from build123d import *

# Parameters (mm, degrees)
SKETCH_W        = 18
SKETCH_H        = 10
PAD_DEPTH       = 17
SKETCH009_R     = 1.5
POCKET_DEPTH    = 4
POCKET001_DEPTH = 2.5
POCKET002_DEPTH = 10.001
SKETCH012_R     = 1.5
POCKET003_DEPTH = 10.001


with BuildPart() as part:
    # Sketch → Pad (new body)
    with BuildSketch(Plane.XY):
        with Locations((9, 5)):
            Rectangle(SKETCH_W, SKETCH_H)
    extrude(amount=PAD_DEPTH)

    # Sketch009 (on DatumPlane) → Pocket (cut, symmetric)
    with BuildSketch(Plane.XY.offset(13)):
        with Locations((3, 5)):
            Circle(SKETCH009_R)
        with Locations((15, 5)):
            Circle(SKETCH009_R)
    extrude(amount=POCKET_DEPTH, both=True, mode=Mode.SUBTRACT)

    # Sketch010 (on DatumPlane) → Pocket001 (cut)
    with BuildSketch(Plane.XY.offset(13)):
        Polygon((4.732051, 2), (6.464102, 5), (4.732051, 8), (1.267949, 8), (0, 8), (0, 2), (1.267949, 2), align=None)
        Polygon((16.732051, 8), (13.267949, 8), (11.535898, 5), (13.267949, 2), (16.732051, 2), (18, 2), (18, 8), align=None)
    extrude(amount=-POCKET001_DEPTH, mode=Mode.SUBTRACT)

    # Sketch011 → Pocket002 (cut, through all)
    with BuildSketch(Plane.XZ):
        Polygon((6.45, 0), (11.55, 0), (13.917136, 4.1), (4.082864, 4.1), align=None)
    extrude(amount=-POCKET002_DEPTH, mode=Mode.SUBTRACT)

    # Sketch012 → Pocket003 (cut, through all)
    with BuildSketch(Plane.XZ):
        with Locations((9, 10)):
            Circle(SKETCH012_R)
    extrude(amount=-POCKET003_DEPTH, mode=Mode.SUBTRACT)


solid = part.part
Design review of the part built by this model. Coordinates are the model's own, in mm. A direction names the side the tool comes from. Coordinates: 2 decimals unless noted, no trailing zeros. Loops run counter-clockwise (first coordinate to the right, second up) from the corner with the lowest first, then second, coordinate; pieces in that order, holes last.
Item 1: Add section A-A (z = 10). Write out the cut boundary in (x, y).
Completed:
outline: (0, 0) - (7.5, 0) - (7.5, 10) - (0, 10) - close; (10.5, 0) - (18, 0) - (18, 10) - (10.5, 10) - close; hole circle Ø3 at (3, 5); hole circle Ø3 at (15, 5)
Item 2: For faces 1 (the flat face through (16.2, 6.4, 13)), 2 (the cylindrical face through (4.386, 4.425, 14.972)), 3 (the flat face through (5.25, 4.93, 2.08)), 4 (the flat face through (1.8, 3.7, 13)), list the 3-axis set-ups (+Z, -Z, +X, -X, +Y, -Y) from which the entire face can be reached by the end or side of a thin tool; tool diameter is ignored.
Completed:
face 1: +X
face 2: +Z
face 3: +Y, -Y
face 4: -X
Item 3: Add section B-B (y = 4.5). Give the number of separate pieces and of enclosed holes in the cut face, and give its area (3 significant figures).
Completed:
separate pieces: 3
enclosed holes: 1
area: 206 mm2
Item 4: Add section C-C (x = 9). Write out the cut boundary in (y, z).
Completed:
outline: (0, 4.1) - (10, 4.1) - (10, 8.5) - (0, 8.5) - close; (0, 11.5) - (10, 11.5) - (10, 17) - (0, 17) - close
Item 5: Add section D-D (z = 12.75). Write out the cut boundary in (x, y), and give its area (3 significant figures).
Completed:
outline: (0, 0) - (18, 0) - (18, 2) - (13.27, 2) - (11.54, 5) - (13.27, 8) - (18, 8) - (18, 10) - (0, 10) - (0, 8) - (4.73, 8) - (6.46, 5) - (4.73, 2) - (0, 2) - close
area: 113 mm2
Item 6: Clearance check with flat-ended pins moving along their axes: pin 1 (1.8 mm diameter, centred on x = 9, z = 10, fed in from -Y); pin 2 (2.5 mm diameter, centred on x = 15, y = 5, fed in from +Z); pin 3 (2 mm diameter, centred on x = 8, y = 8, fed in from -Z). State where each tip first meets the part, or that it passes through.
Completed:
pin 1: passes through
pin 2: stops at z = 9
pin 3: stops at z = 4.1
Item 7: Wall thickness on L1, parallel to Y at x = 15, z = 9.85; L2, parallel to Z at x = 12.75, y = 5.75; L3, parallel to Z at x = 2.5, y = 7.25: over which ranges is each line inside the solid? List them lowest first.
Completed:
L1: y = 0 to 3.5, 6.5 to 10
L2: z = 0 to 2.08, 4.1 to 10.5, 13 to 17
L3: z = 0 to 10.5, 13 to 17
Item 8: Draft analysis for pull direction Z (two halves, no side actions). For faces 5 (the flat face through (3, 5, 9)), 6 (the flat face through (9, 5, 4.1)), 7 (the cylindrical face through (13.5, 5.07, 15.03)), 8 (the flat face through (12.717, 4.93, 2.021)), state which applies: pulls with the +Z half, pulls with the -Z half, needs draft (parallel to the pull), parting line crosses it, or undercut.
Completed:
face 5: pulls with the +Z half
face 6: undercut
face 7: needs draft
face 8: undercut
